Here's how the part is built. I have some questions about the finished solid (model axes, mm). Coordinates: 2 decimals unless noted, no trailing zeros. Write each loop counter-clockwise with the first axis right and the second up, starting at its lowest first coordinate (ties: lowest second). Pieces come first, ordered by that corner, then holes.
Item 1: We'd pull the mould along X, two halves only. Please class faces 1 (the face through (177, -2, 0)), 2 (the face through (-3.895, 3.105, 1.615)), 3 (the face through (-180, 0, 0)): +X half, -X half, draft (parallel to the pull), parting line (faces both ways), or undercut.
Item 2: If I drill on line 1 (X direction, y = 2.75, z = -0.5); line 2 (Z direction, x = 45.5, y = -0.5); line 3 (Z direction, x = -114, y = -1), over which ranges is the centre line in solid material (lowest first)?
Item 3: I'm going to push flat-ended pins straight in: pin 1 Ø4 at (x, z) = (95, -2.5) entering from -Y; pin 2 Ø3 at (x, z) = (-67.5, -2) entering from +Y; pin 3 Ø1 at (x, y) = (126.5, -1.5) entering from -Z. Where does each tip first touch, or does it pass through?
Item 4: If we section it at A-A (x = -82): Please give me the cut outline in (y, z).
from build123d import *

# Parameters (mm, degrees)
FILLET1_R = 0.2
FILLET2_R = 0.2
FILLET3_R = 0.4


with BuildPart() as part:
    # Sketch1 → Revolve1 (revolve)
    with BuildSketch(Plane.XY, mode=Mode.PRIVATE) as revolve1_sk:
        Polygon((-180, 0), (180, 0), (180, 2.9), (178.5, 2.9), (178.5, 1.5), (177, 1.5), (177, 3.5), (-180, 3.5), align=None)
    revolve(revolve1_sk.sketch.rotate(Axis((-180, 0, 0), (1, 0, 0)), 90), axis=Axis((-180, 0, 0), (1, 0, 0)))

    # Fillet1
    fillet1_edges = [part.edges().sort_by_distance(p)[0] for p in [
        (177, 0, -3.5),
    ]]
    fillet(fillet1_edges, radius=FILLET1_R)

    # Fillet2
    fillet2_edges = [part.edges().sort_by_distance(p)[0] for p in [
        (180, 0, -2.9),
        (178.5, 0, -2.9),
    ]]
    fillet(fillet2_edges, radius=FILLET2_R)

    # Fillet3
    fillet3_edges = [part.edges().sort_by_distance(p)[0] for p in [
        (-180, 0, -3.5),
    ]]
    fillet(fillet3_edges, radius=FILLET3_R)


solid = part.part
Answer list:
1. face 1: undercut
1. face 2: draft
1. face 3: -X half
2. line 1: x = -180 to 177, 178.52 to 179.98
2. line 2: z = -3.46 to 3.46
2. line 3: z = -3.35 to 3.35
3. pin 1: stops at y = -3.46
3. pin 2: stops at y = 3.46
3. pin 3: stops at z = -3.35
4. outline: circle Ø7 at (0, 0)
